from build123d import *

# Parameters (mm, degrees)
CROQUIS1_R              = 22.5
SALIENTE_EXTRUIR1_DEPTH = 60
CROQUIS2_R              = 7.5
SALIENTE_EXTRUIR2_DEPTH = 5


with BuildPart() as part:
    # Croquis1 → Saliente-Extruir1 (new body)
    with BuildSketch(Plane(origin=(0, 0, 0), x_dir=(1, 0, 0), z_dir=(0, 1, 0))):
        with BuildLine():
            Line((-29.464610793, 5.64240293), (-29.464610793, -5.64240293))
            ThreePointArc((-29.464610793, -5.64240293), (0, -30), (29.464610793, -5.64240293))
            Line((29.464610793, -5.64240293), (29.464610793, 5.64240293))
            ThreePointArc((29.464610793, 5.64240293), (0, 30), (-29.464610793, 5.64240293))
        make_face()
        with Locations(Location((0, 0, 0), (0, 0, 270))):  # turned: the seam where the file's is
            Circle(CROQUIS1_R, mode=Mode.SUBTRACT)
    extrude(amount=SALIENTE_EXTRUIR1_DEPTH)

    # Croquis2 → Saliente-Extruir2 (add, symmetric)
    with BuildSketch(Plane.XY):
        with BuildLine():
            Line((29.464610793, 60), (29.464610793, 0))
            Line((29.464610793, 0), (49.359858197, 0))
            ThreePointArc((49.359858197, 0), (55.675693274, 2.246921433), (59.153291312, 7.977954546))
            Line((59.153291312, 7.977954546), (83.929633957, 127.977954546))
            ThreePointArc((83.929633957, 127.977954546), (81.889279409, 136.315835078), (74.136200842, 140))
            Line((74.136200842, 140), (61.411819936, 140))
            ThreePointArc((61.411819936, 140), (54.340752124, 137.071067812), (51.411819936, 130))
            Line((51.411819936, 130), (51.411819936, 70))
            ThreePointArc((51.411819936, 70), (48.482887748, 62.928932188), (41.411819936, 60))
            Line((41.411819936, 60), (29.464610793, 60))
        make_face()
        with Locations((45, 19.203564165)):
            Circle(CROQUIS2_R, mode=Mode.SUBTRACT)
        with Locations(Location((66.411819936, 123.15179788, 0), (0, 0, 180))):  # turned: the seam where the file's is
            Circle(CROQUIS2_R, mode=Mode.SUBTRACT)
        with BuildLine():
            Line((-39.648553202, 61.179498685), (-27.706402099, 60.831887788))
            Line((-27.706402099, 60.831887788), (-29.452136484, 0.857289737))
            Line((-29.452136484, 0.857289737), (-49.33896092, 1.436153362))
            ThreePointArc((-49.33896092, 1.436153362), (-55.586746623, 3.865886366), (-58.896124671, 9.695675863))
            Line((-58.896124671, 9.695675863), (-80.17050909, 130.365753854))
            ThreePointArc((-80.17050909, 130.365753854), (-77.888422947, 138.640739128), (-70.031433878, 142.097764037))
            Line((-70.031433878, 142.097764037), (-57.31244004, 141.727540882))
            ThreePointArc((-57.31244004, 141.727540882), (-50.329584837, 138.594111934), (-47.607629428, 131.44081881))
            Line((-47.607629428, 131.44081881), (-49.353363814, 71.466220758))
            ThreePointArc((-49.353363814, 71.466220758), (-46.631408405, 64.312927634), (-39.648553202, 61.179498685))
        make_face()
        with Locations((-62.800531307, 125.03194958)):
            Circle(CROQUIS2_R, mode=Mode.SUBTRACT)
        with Locations(Location((-44.422209834, 20.504734822, 0), (0, 0, 180))):  # turned: the seam where the file's is
            Circle(CROQUIS2_R, mode=Mode.SUBTRACT)
    extrude(amount=SALIENTE_EXTRUIR2_DEPTH, both=True)


solid = part.part
Verification items for the finished model (mm, model axes). A direction names the side the tool comes from. Coordinates: 2 decimals unless noted, no trailing zeros. Order: outer loops, then holes, each group sorted by start corner. A loop starts at its lowest first (then second) coordinate and runs counter-clockwise, first axis right, second up. Notation, with made-up numbers: M 36,-12.75 L 43,-12.75 A23 cw 43,1.25 Z; hole C 9,2.5 d9. An arc over 180 degrees is marked long. Return JSON: item names as keys, results as strings.
1) Cross-section at D-D, the plane y = 47.5. Record the boundary of the cut face in (x, z).
Answer list:
{"outline": "M -65.56,-5 L -29.46,-5 L -29.46,-5.64 A30 ccw 29.46,-5.64 L 29.46,-5 L 67.31,-5 L 67.31,5 L 29.46,5 L 29.46,5.64 A30 ccw -29.46,5.64 L -29.46,5 L -65.56,5 Z; hole C 0,0 d45"}
2) Release check for a two-part mould opening along Z. For faces 4 (the cylindrical face through (-8.618, 29.58, 20.784)), 5 (the cylindrical face through (52.154, 21.456, -0.07)), 6 (the flat face through (56, 71, -5)), 7 (the flat face through (56, 71, 5)) record: +Z half, -Z half, draft (parallel to the pull), parting line (faces both ways), or undercut.
Answer list:
{"face 4": "undercut", "face 5": "draft", "face 6": "-Z half", "face 7": "+Z half"}
3) Gauge pin test, flat ends, axial feed: pin 1 (0.7 mm diameter, centred on y = 34, z = 5, fed in from +X); pin 2 (11 mm diameter, centred on y = 98, z = 2, fed in from -X); pin 3 (24 mm diameter, centred on x = -44.42, y = 20.5, fed in from -Z). Record the tip position at first contact, or that the pin passes through.
Answer list:
{"pin 1": "x = 64.6", "pin 2": "x = -75.43", "pin 3": "z = -5"}
4) Cross-section at C-C, the plane x = -8. Record the boundary of the cut face in (y, z), and give its area (3 significant figures).
Answer list:
{"outline": "M 0,-28.91 L 60,-28.91 L 60,-21.03 L 0,-21.03 Z; M 0,21.03 L 60,21.03 L 60,28.91 L 0,28.91 Z", "area": "946 mm2"}
5) Cross-section at A-A, the plane z = 0. Record the boundary of the cut face in (x, y), and give its area (3 significant figures).
Answer list:
{"outline": "M -80.17,130.37 L -58.9,9.7 A10 ccw -49.34,1.44 L -29.46,0.86 L -29.46,0 L -22.5,0 L -22.5,60 L -27.73,60 L -27.71,60.83 L -39.65,61.18 A10 cw -49.35,71.47 L -47.61,131.44 A10 ccw -57.31,141.73 L -70.03,142.1 A10 ccw Z; M 22.5,0 L 49.36,0 A10 ccw 59.15,7.98 L 83.93,127.98 A10 ccw 74.14,140 L 61.41,140 A10 ccw 51.41,130 L 51.41,70 A10 cw 41.41,60 L 22.5,60 Z; hole C -62.8,125.03 d15; hole C -44.42,20.5 d15; hole C 45,19.2 d15; hole C 66.41,123.15 d15", "area": "8,370 mm2"}
6) Access from +Z, -Z, +X, -X, +Y, -Y to the whole of each face (thin tool, end or side, straight path). Record for faces 1 (the cylindrical face through (54.42, 137.15, -0.07)), 2 (the flat face through (68, 140, 0)), 3 (the cylindrical face through (-46.706, 64.393, 0.07)).
Answer list:
{"face 1": "+Z, -Z, +Y", "face 2": "+Z, -Z, +X, +Y", "face 3": "+Z, -Z"}
7) Thickness scan on L1, parallel to Z at x = -51, y = 14.5; L2, parallel to X at y = 15, z = -2.5; L3, parallel to X at y = 35, z = 0. Record the ranges inside material, lowest first. Write a range as [from, to].
Answer list:
{"L1": "[-5, 5]", "L2": "[-59.83, -49.52], [-39.33, -22.36], [22.36, 38.79], [51.21, 60.6]", "L3": "[-63.36, -22.5], [22.5, 64.73]"}
8) Cross-section at B-B, the plane y = 64.5. Record the boundary of the cut face in (x, z).
Answer list:
{"outline": "M -68.56,-5 L -46.8,-5 L -46.8,5 L -68.56,5 Z; M 49.76,-5 L 70.82,-5 L 70.82,5 L 49.76,5 Z"}
